Work out the finished part from the listing and answer in its coordinate system (mm). Face numbers are marked on the shaded views. A direction names the side the tool comes from. Coordinates: 2 decimals unless noted, no trailing zeros. Loops run counter-clockwise (first coordinate to the right, second up) from the corner with the lowest first, then second, coordinate; pieces in that order, holes last. Notation, with made-up numbers: (16.25, 8.5) -> (25.25, 8.5) arc R23 cw to (25.25, 18.5) -> close; hole circle Ø4 at (-32.75, 64.5). An arc over 180 degrees is marked (long way). Use a Markdown table: item, result.
from build123d import *

# Parameters (mm, degrees)
F0_R     = 9.9949
F0_R_2   = 6.3373
F1_DEPTH = 19.5072
F0_R_3   = 29.5402
F0_R_4   = 8.001
F2_DEPTH = 7.874
F0_R_5   = 35.0012
F3_DEPTH = 15.0114


with BuildPart() as f1:
    # F0 (on Front) → F1 (new body)
    with BuildSketch(Plane.XZ):
        Circle(F0_R)
        Circle(F0_R_2, mode=Mode.SUBTRACT)
    extrude(amount=F1_DEPTH)

    # F0 (on Front) → F2 (join)
    with BuildSketch(Plane.XZ):
        Circle(F0_R_3)
        with Locations((-2.421228, -19.275159)):
            Circle(F0_R_4, mode=Mode.SUBTRACT)
        with Locations((19.409321, -2.979115)):
            Circle(F0_R_4, mode=Mode.SUBTRACT)
        with Locations((-19.332217, 3.170335)):
            Circle(F0_R_4, mode=Mode.SUBTRACT)
        Circle(F0_R, mode=Mode.SUBTRACT)
        with Locations((3.728223, 19.158907)):
            Circle(F0_R_4, mode=Mode.SUBTRACT)
    extrude(amount=F2_DEPTH)

    # F0 (on Front) → F3 (join)
    with BuildSketch(Plane.XZ):
        Circle(F0_R_5)
        Circle(F0_R_3, mode=Mode.SUBTRACT)
    extrude(amount=F3_DEPTH)


solid = f1.part
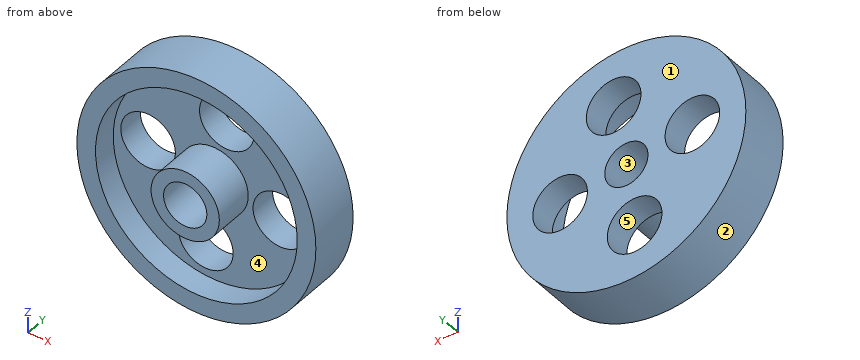
Q1. For the marked faces 4 and 5, determine the directions among +Z, -Z, +X, -X, +Y, -Y from which every point of the face is accessible in a straight line to the end or side of a thin tool.
Solved:
| item | result |
|---|---|
| face 4 | -Y |
| face 5 | +Y, -Y |
Q2. Section B-B on y = -11 is taken. Determine the outline of the cut face in (x, z).
Solved:
| item | result |
|---|---|
| outline | circle Ø70 at (0, 0); circle Ø19.99 at (0, 0); hole circle Ø59.08 at (0, 0); hole circle Ø12.67 at (0, 0) |
Q3. Section A-A on x = 0 is taken. Determine the outline of the cut face in (y, z), and give its area (3 significant figures).
Solved:
| item | result |
|---|---|
| outline | (-19.51, -9.99) -> (-7.87, -9.99) -> (-7.87, -11.65) -> (0, -11.65) -> (0, -6.34) -> (-19.51, -6.34) -> close; (-19.51, 6.34) -> (0, 6.34) -> (0, 12.08) -> (-7.87, 12.08) -> (-7.87, 9.99) -> (-19.51, 9.99) -> close; (-15.01, -35) -> (0, -35) -> (0, -26.9) -> (-7.87, -26.9) -> (-7.87, -29.54) -> (-15.01, -29.54) -> close; (-15.01, 29.54) -> (-7.87, 29.54) -> (-7.87, 26.24) -> (0, 26.24) -> (0, 35) -> (-15.01, 35) -> close |
| area | 383 mm² |
Q4. Section C-C on z = 0 is taken. Determine the outline of the cut face in (x, y).
Solved:
| item | result |
|---|---|
| outline | (-35, -15.01) -> (-29.54, -15.01) -> (-29.54, -7.87) -> (-26.68, -7.87) -> (-26.68, 0) -> (-35, 0) -> close; (-11.99, -7.87) -> (-9.99, -7.87) -> (-9.99, -19.51) -> (-6.34, -19.51) -> (-6.34, 0) -> (-11.99, 0) -> close; (6.34, -19.51) -> (9.99, -19.51) -> (9.99, -7.87) -> (11.98, -7.87) -> (11.98, 0) -> (6.34, 0) -> close; (26.84, -7.87) -> (29.54, -7.87) -> (29.54, -15.01) -> (35, -15.01) -> (35, 0) -> (26.84, 0) -> close |
Q5. Section D-D on x = -18 is taken. Determine the outline of the cut face in (y, z).
Solved:
| item | result |
|---|---|
| outline | (-15.01, -30.02) -> (0, -30.02) -> (0, -4.72) -> (-7.87, -4.72) -> (-7.87, -23.42) -> (-15.01, -23.42) -> close; (-15.01, 23.42) -> (-7.87, 23.42) -> (-7.87, 11.06) -> (0, 11.06) -> (0, 30.02) -> (-15.01, 30.02) -> close |
Q6. Given pin 1 Ø4 at (x, y) = (2, -14.5) entering from +Z; pin 2 Ø2 at (x, z) = (-25, -17.5) entering from -Y; pin 3 Ø2 at (x, y) = (12, -11) entering from +Z, each flat-ended and moving along its own axis, determine where each tip first touches the part or whether it passes through.
Solved:
| item | result |
|---|---|
| pin 1 | z = 35 |
| pin 2 | y = -15.01 |
| pin 3 | z = 33.23 |
Q7. Consider line 1 (Z direction, x = 0, y = -10.5); line 2 (Z direction, x = -8, y = -9); line 3 (X direction, y = -3.5, z = 2.5). Determine where each line is inside the solid, lowest interval first. Write a range as [from, to].
Solved:
| item | result |
|---|---|
| line 1 | [-35, -29.54], [-9.99, -6.34], [6.34, 9.99], [29.54, 35] |
| line 2 | [-34.07, -28.44], [-5.99, 5.99], [28.44, 34.07] |
| line 3 | [-34.91, -27.31], [-11.36, -5.82], [5.82, 13.58], [25.24, 34.91] |
Q8. Determine the mould class of the marked faces 1, 2 and 3 for opening direction X: pulls with the +X half, pulls with the -X half, needs draft (parallel to the pull), parting line crosses it, or undercut.
Solved:
| item | result |
|---|---|
| face 1 | needs draft |
| face 2 | parting line crosses it |
| face 3 | undercut |
